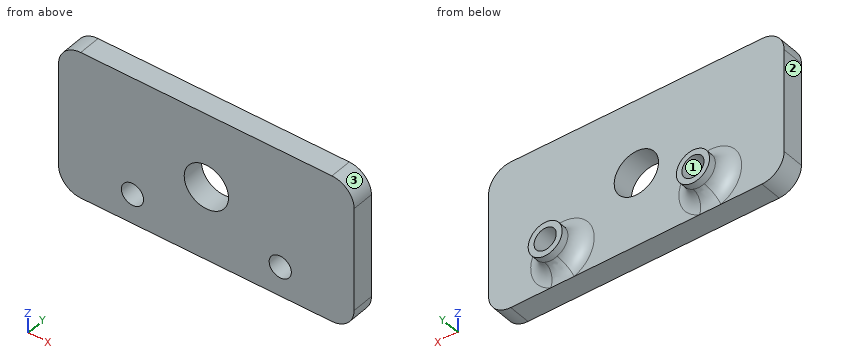
from build123d import *

# Parameters (mm, degrees)
SKETCH1_W           = 40
SKETCH1_H           = 20
SKETCH1_R           = 1.5
BOSS_EXTRUDE1_DEPTH = 3
FILLET1_R           = 3
SKETCH2_R           = 2.25
SKETCH2_R_2         = 1.5
SKETCH2_R_3         = 2.3
BOSS_EXTRUDE2_DEPTH = 3
SKETCH3_R           = 3
CUT_EXTRUDE1_DEPTH  = 10
FILLET2_R           = 2


with BuildPart() as part:
    # Sketch1 → Boss-Extrude1 (new body)
    with BuildSketch(Plane(origin=(0, 0, 0), x_dir=(1, 0, 0), z_dir=(0, 1, 0))):
        Rectangle(SKETCH1_W, SKETCH1_H)
        with Locations(Location((-10, 6, 0), (0, 0, 270))):
            Circle(SKETCH1_R, mode=Mode.SUBTRACT)
        with Locations(Location((10, 6, 0), (0, 0, 90))):
            Circle(SKETCH1_R, mode=Mode.SUBTRACT)
    extrude(amount=BOSS_EXTRUDE1_DEPTH)

    # Fillet1
    fillet1_edges = [part.edges().sort_by_distance(p)[0] for p in [
        (20, 1.5, 10),
        (-20, 1.5, 10),
        (-20, 1.5, -10),
        (20, 1.5, -10),
    ]]
    fillet(fillet1_edges, radius=FILLET1_R)

    # Sketch2 → Boss-Extrude2 (add)
    # profile 1 of 2: a face of its own
    with BuildSketch(Plane(origin=(0, 3, 0), x_dir=(1, 0, 0), z_dir=(0, 1, 0))):
        with Locations(Location((-10, 6, 0), (0, 0, 270))):
            Circle(SKETCH2_R)
        with Locations(Location((-10, 6, 0), (0, 0, 270))):
            Circle(SKETCH2_R_2, mode=Mode.SUBTRACT)
    # profile 2 of 2: a face of its own
    with BuildSketch(Plane(origin=(0, 3, 0), x_dir=(1, 0, 0), z_dir=(0, 1, 0))):
        with Locations(Location((10, 6, 0), (0, 0, 270))):
            Circle(SKETCH2_R_3)
        with Locations(Location((10, 6, 0), (0, 0, 90))):
            Circle(SKETCH2_R_2, mode=Mode.SUBTRACT)
    extrude(amount=BOSS_EXTRUDE2_DEPTH)

    # Sketch3 → Cut-Extrude1 (cut)
    with BuildSketch(Plane(origin=(0, 3, 0), x_dir=(1, 0, 0), z_dir=(0, 1, 0))):
        with Locations(Location((0, 0, 0), (0, 0, 270))):
            Circle(SKETCH3_R)
    extrude(amount=-CUT_EXTRUDE1_DEPTH, mode=Mode.SUBTRACT)

    # Fillet2
    fillet2_edges = [part.edges().sort_by_distance(p)[0] for p in [
        (-10, 3, -8.25),
        (10, 3, -8.3),
    ]]
    fillet(fillet2_edges, radius=FILLET2_R)


solid = part.part
Input: part model. Units: mm. Frame: model coordinates. Face numbers are marked on the shaded views. Give positions to 0.01 mm unless a question says otherwise; leave off trailing zeros. Write each loop counter-clockwise with the first axis right and the second up, starting at its lowest first coordinate (ties: lowest second). Pieces come first, ordered by that corner, then holes.
Q1. First-contact query: P1, Ø1.5, axis at x = -13, z = -0.5, coming from the +Y side; P2, Ø2.5, axis at x = -10, z = -6, coming from the +Y side. Flat tips, straight axial feed; report the tip coordinate or a pass-through.
Q2. Section C-C, the plane x = 0. Output: boundary loops of the cut face in (y, z).
Q3. Section D-D, the plane z = -6. Output: boundary loops of the cut face in (x, y), plus the area to 3 significant figures.
Q4. Section B-B, the plane y = 2.5. Output: boundary loops of the cut face in (x, z).
Q5. Material intervals for probe 1 along X at (y, z) = (1.95, -6); probe 2 along X at (y, z) = (0.8, 0); probe 3 along Y at (x, z) = (-7.5, 8), sorted ascending.
Q6. Section A-A, the plane z = 0. Output: boundary loops of the cut face in (x, y).
Q7. Pull-direction query (Z, two-part tool) for the marked faces 1, 2 and 3; classes: pulls with the +Z half, pulls with the -Z half, needs draft (parallel to the pull), parting line crosses it, or undercut.
Filled in:
1. P1: stops at y = 3
1. P2: passes through
2. outline: (0, -10) - (3, -10) - (3, -3) - (0, -3) - close; (0, 3) - (3, 3) - (3, 10) - (0, 10) - close
3. outline: (-20, 0) - (-11.5, 0) - (-11.5, 6) - (-12.25, 6) - (-12.25, 5) arc R2 cw to (-14.25, 3) - (-20, 3) - close; (-8.5, 0) - (8.5, 0) - (8.5, 6) - (7.7, 6) - (7.7, 5) arc R2 cw to (5.7, 3) - (-5.75, 3) arc R2 cw to (-7.75, 5) - (-7.75, 6) - (-8.5, 6) - close; (11.5, 0) - (20, 0) - (20, 3) - (14.3, 3) arc R2 cw to (12.3, 5) - (12.3, 6) - (11.5, 6) - close
3. area: 115 mm2
4. outline: (-20, -7) arc R3 ccw to (-17, -10) - (17, -10) arc R3 ccw to (20, -7) - (20, 7) arc R3 ccw to (17, 10) - (-17, 10) arc R3 ccw to (-20, 7) - close; hole circle Ø3 at (-10, -6); hole circle Ø6 at (0, 0); hole circle Ø3 at (10, -6)
5. probe 1: x = -20 to -11.5, -8.5 to 8.5, 11.5 to 20
5. probe 2: x = -20 to -3, 3 to 20
5. probe 3: y = 0 to 3
6. outline: (-20, 0) - (-3, 0) - (-3, 3) - (-20, 3) - close; (3, 0) - (20, 0) - (20, 3) - (3, 3) - close
7. face 1: undercut
7. face 2: needs draft
7. face 3: pulls with the +Z half
